Work out the finished part from the listing and answer in its coordinate system (mm). A direction names the side the tool comes from. Round coordinates to 2 decimals unless told otherwise and drop trailing zeros. Write each loop counter-clockwise with the first axis right and the second up, starting at its lowest first coordinate (ties: lowest second). Pieces come first, ordered by that corner, then holes.
1. Find section B-B (x = 30.25). Write down the section's boundary in (y, z).
2. Find section A-A (y = -12.5). Write down the section's boundary in (x, z).
3. Determine the mould class of faces 5 (the face through (22.882, 0, -6)), 6 (the face through (24.403, 23.824, 24.511)), 7 (the face through (28.997, -10.575, -25.805)), 8 (the face through (24.403, -23.926, 24.42)) for opening direction Y: pulls with the +Y half, pulls with the -Y half, needs draft (parallel to the pull), parting line crosses it, or undercut.
4. Find section C-C (z = -4). Write down the section's boundary in (x, y).
5. Find section D-D (y = 10). Count the separate pieces of the cut face and the enclosed holes in it, and give its area (3 significant figures).
6. A tool of negligible diameter and unlimited length cuts with its end or side. For faces 1 (the face through (31.91, 5.888, 19.328)), 2 (the face through (32, 0, -24.284)), 3 (the face through (24.4, 20.54, 21.81)), 4 (the face through (28.84, 21.995, 12.402)), from which of +Z, -Z, +X, -X, +Y, -Y can it reach the whole face along a straight path? Write none if from no direction.
7. Straight lines are drawn through the part: probe 1 along Z at (x, y) = (28.75, 12.5); probe 2 along Z at (x, y) = (37.25, 6); probe 3 along Y at (x, z) = (25.5, 19). For each, find the intervals that lie inside material, in ascending order.
8. Flat-ended cylindrical pins translate along their axes: pin 1 Ø15.5 at (y, z) = (-13.5, 14) entering from +X; pin 2 Ø1.8 at (x, y) = (30.38, 10) entering from -Z; pin 3 Ø3 at (x, y) = (32, -5) entering from +Z; pin 4 Ø10 at (y, z) = (12.5, 12.72) entering from +X. Find the tip coordinate at first contact, or state that the pin passes through.
```python
from build123d import *

# Parameters (mm, degrees)
EXTRUDE_1_DEPTH     = 27.5
SKETCH_3_R          = 0.75
CUT_EXTRUDE_3_DEPTH = 3
REVOLVE_1_ANGLE     = 270
SKETCH_2_R          = 1.5
CUT_EXTRUDE_4_DEPTH = 3


with BuildPart() as part:
    # 草图1 → 凸台-拉伸1 (new, symmetric)
    with BuildSketch(Plane(origin=(0, 0, 0), x_dir=(1, 0, 0), z_dir=(0, 1, 0))):
        Polygon((22.882352941, -27.715686275), (25.882352941, -27.715686275), (25.882352941, 24.284313725), (37.882352941, 24.284313725), (37.882352941, 27.284313725), (22.882352941, 27.284313725), align=None)
    extrude(amount=EXTRUDE_1_DEPTH, both=True)

    # 草图3 → 切除-拉伸3 (cut)
    with BuildSketch(Plane(origin=(25.882352941, 0, 0), x_dir=(0, 0, -1), z_dir=(1, 0, 0))):
        with BuildLine():
            Line((-19.394463571, 5.743970558), (-19.394463571, -5.743970558))
            Line((-19.394463571, -5.743970558), (-18.726093915, -6.48959236))
            ThreePointArc((-18.726093915, -6.48959236), (-12.715686275, -21), (-6.705278634, -6.48959236))
            Line((-6.705278634, -6.48959236), (-6.036908978, -5.743970558))
            ThreePointArc((-6.036908978, -5.743970558), (-4.017201465, 0), (-6.036908978, 5.743970558))
            Line((-6.036908978, 5.743970558), (-6.705278634, 6.48959236))
            ThreePointArc((-6.705278634, 6.48959236), (-12.715686275, 21), (-18.726093915, 6.48959236))
            Line((-18.726093915, 6.48959236), (-19.394463571, 5.743970558))
        make_face()
        Polygon((-21.215686275, 27.5), (-27.715686275, 27.5), (-27.715686275, 20.24982538), align=None)
        Polygon((-21.215686275, -27.5), (-27.715686275, -20.24982538), (-27.715686275, -27.5), align=None)
        with Locations((-4.215686275, -21)):
            Circle(SKETCH_3_R)
        with Locations((-21.215686275, -21)):
            Circle(SKETCH_3_R)
        with Locations((-4.215686275, 21)):
            Circle(SKETCH_3_R)
        with Locations((-21.215686275, 21)):
            Circle(SKETCH_3_R)
    extrude(amount=-CUT_EXTRUDE_3_DEPTH, mode=Mode.SUBTRACT)

    # 草图5 → 旋转1 (revolve, symmetric)
    with BuildSketch(Plane(origin=(0, 0, 12.715686275), x_dir=(0, -1, 0), z_dir=(0, 0, 1))) as revolve_1_sk:
        Polygon((-22, 25.882352941), (-21, 25.882352941), (-21, 31.882352941), (-23.5, 37.882352941), (-24.5, 37.882352941), (-22, 31.882352941), align=None)
    revolve_1 = revolve(axis=Axis((32.882352941, 12.5, 12.715686275), (-1, 0, 0)), revolution_arc=REVOLVE_1_ANGLE / 2)
    revolve_1 = revolve_1 + revolve(revolve_1_sk.sketch, axis=Axis((32.882352941, 12.5, 12.715686275), (1, 0, 0)), revolution_arc=REVOLVE_1_ANGLE / 2)

    # 镜向1: 旋转1 across plane
    add(revolve_1.mirror(Plane.ZX))

    # 草图2 → 切除-拉伸4 (cut)
    with BuildSketch(Plane(origin=(0, 0, -27.284313725), x_dir=(-1, 0, 0), z_dir=(0, 0, -1))):
        with Locations((-30.382352941, 10)):
            Circle(SKETCH_2_R)
        with Locations((-30.382352941, -10)):
            Circle(SKETCH_2_R)
    extrude(amount=-CUT_EXTRUDE_4_DEPTH, mode=Mode.SUBTRACT)


solid = part.part
```
Worked answers:
1. outline: (-27.5, -27.28) - (-11.49, -27.28) - (-11.49, -24.28) - (-27.5, -24.28) - close; (-8.51, -27.28) - (8.51, -27.28) - (8.51, -24.28) - (-8.51, -24.28) - close; (-6.49, 6.71) arc R8.5 cw (long way) to (-6.49, 18.73) - (-5.78, 19.43) arc R9.5 ccw (long way) to (-5.78, 6) - close; (5.78, 6) arc R9.5 ccw (long way) to (5.78, 19.43) - (6.49, 18.73) arc R8.5 cw (long way) to (6.49, 6.71) - close; (11.49, -27.28) - (27.5, -27.28) - (27.5, -24.28) - (11.49, -24.28) - close
2. outline: (22.88, -27.28) - (37.88, -27.28) - (37.88, -24.28) - (25.88, -24.28) - (25.88, 3.22) - (31.88, 3.22) - (37.88, 0.72) - (37.88, 1.72) - (31.88, 4.22) - (22.88, 4.22) - close; (22.88, 21.22) - (31.88, 21.22) - (37.88, 23.72) - (37.88, 24.72) - (31.88, 22.22) - (25.88, 22.22) - (25.88, 27.72) - (22.88, 27.72) - close
3. face 5: needs draft
3. face 6: pulls with the +Y half
3. face 7: undercut
3. face 8: pulls with the -Y half
4. outline: (22.88, -27.5) - (25.88, -27.5) - (25.88, 27.5) - (22.88, 27.5) - close
5. separate pieces: 3
5. enclosed holes: 0
5. area: 168 mm2
6. face 1: +X
6. face 2: +X, +Y, -Y
6. face 3: -X
6. face 4: none
7. probe 1: z = -27.28 to -24.28, 3.22 to 4.22, 21.22 to 22.22
7. probe 2: z = -27.28 to -24.28, 2.94 to 4.17, 21.26 to 22.49
7. probe 3: y = -27.5 to -18.22, -6.78 to -6.18, 6.18 to 6.78, 18.22 to 27.5
8. pin 1: stops at x = 33.99
8. pin 2: stops at z = 3.35
8. pin 3: stops at z = 20.39
8. pin 4: passes through
